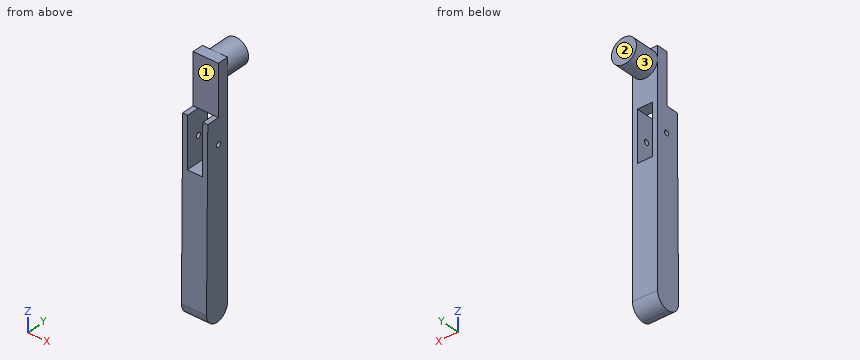
from build123d import *

# Parameters (mm, degrees)
BOSS_EXTRUDE1_DEPTH = 50
BOSS_EXTRUDE2_START = 35.418994
SKETCH2_R           = 25
BOSS_EXTRUDE2_DEPTH = 50
SKETCH4_W           = 30
SKETCH4_H           = 100
CUT_EXTRUDE1_DEPTH  = 318.853328976
SKETCH5_R           = 5
CUT_EXTRUDE2_DEPTH  = 326.310841007


with BuildPart() as part:
    # Sketch1 → Boss-Extrude1 (new body)
    with BuildSketch(Plane(origin=(0, 0, 0), x_dir=(0, 0, -1), z_dir=(1, 0, 0))):
        with BuildLine():
            Line((140.111731844, 35.418994413), (-209.888268156, 35.418994413))
            Line((-209.888268156, 35.418994413), (-309.888268156, 35.418994413))
            Line((-309.888268156, 35.418994413), (-309.888268156, 13.43575419))
            Line((-309.888268156, 13.43575419), (-209.888268156, 13.43575419))
            Line((-209.888268156, 13.43575419), (-209.888268156, -11.56424581))
            Line((-209.888268156, -11.56424581), (139.680798176, -14.577291234))
            ThreePointArc((139.680798176, -14.577291234), (115.112660449, 10.634469251), (140.111731844, 35.418994413))
        make_face()
        with BuildLine():
            Line((140.111731844, -14.581005587), (140.111731844, 35.418994413))
            ThreePointArc((140.111731844, 35.418994413), (115.112660449, 10.634469251), (139.680798176, -14.577291234))
            Line((139.680798176, -14.577291234), (140.111731844, -14.581005587))
        make_face()
        with BuildLine():
            ThreePointArc((165.111731844, 10.418994413), (157.789401373, 28.096663943), (140.111731844, 35.418994413))
            Line((140.111731844, 35.418994413), (140.111731844, -14.581005587))
            ThreePointArc((140.111731844, -14.581005587), (157.789401373, -7.258675116), (165.111731844, 10.418994413))
        make_face()
    extrude(amount=BOSS_EXTRUDE1_DEPTH)

    # Sketch2 → Boss-Extrude2 (add)
    with BuildSketch(Plane(origin=(0, 0, 0), x_dir=(1, 0, 0), z_dir=(0, 1, 0)).offset(BOSS_EXTRUDE2_START)):
        with Locations(Location((25, -284.888268156, 0), (0, 0, 270))):
            Circle(SKETCH2_R)
    extrude(amount=BOSS_EXTRUDE2_DEPTH)

    # Sketch4 → Cut-Extrude1 (cut, through all)
    with BuildSketch(Plane(origin=(0, 35.418994413, 0), x_dir=(1, 0, 0), z_dir=(0, 1, 0))):
        with Locations((25, -159.888268156)):
            Rectangle(SKETCH4_W, SKETCH4_H)
    extrude(amount=-CUT_EXTRUDE1_DEPTH, mode=Mode.SUBTRACT)

    # Sketch5 → Cut-Extrude2 (cut, through all)
    with BuildSketch(Plane(origin=(50, 0, 0), x_dir=(0, 0, -1), z_dir=(1, 0, 0))):
        with Locations((-159.888268156, 13.945126907)):
            Circle(SKETCH5_R)
    extrude(amount=-CUT_EXTRUDE2_DEPTH, mode=Mode.SUBTRACT)


solid = part.part
Geometry check sheet. Reference: the model listing, model coordinates, mm. Face numbers are marked on the shaded views. A direction names the side the tool comes from. Give positions to 0.01 mm unless a question says otherwise; leave off trailing zeros. Write each loop counter-clockwise with the first axis right and the second up, starting at its lowest first coordinate (ties: lowest second). Pieces come first, ordered by that corner, then holes.
1) Go/stop test with flat-tipped pins: pin 1 Ø25 at (x, z) = (37.5, 257) entering from -Y; pin 2 Ø6 at (x, y) = (15.5, 57) entering from -Z; pin 3 Ø5 at (x, y) = (45.5, 0.5) entering from +Z. Record where each tip stops, or that it passes through.
Values follow:
pin 1: stops at y = 13.44
pin 2: stops at z = 260.75
pin 3: stops at z = 209.89
2) Cross-section at B-B (x = 5). Record the boundary of the cut face in (y, z).
Values follow:
outline: (-14.58, -140.11) arc R25 ccw to (35.42, -140.11) - (35.42, 269.89) - (85.42, 269.89) - (85.42, 299.89) - (35.42, 299.89) - (35.42, 309.89) - (13.44, 309.89) - (13.44, 209.89) - (-11.56, 209.89) - close; hole circle Ø10 at (13.95, 159.89)
3) Cross-section at C-C (y = 48). Record the boundary of the cut face in (x, z).
Values follow:
outline: circle Ø50 at (25, 284.89)
4) Cross-section at D-D (z = 13). Record the boundary of the cut face in (x, y), plus the area to 3 significant figures.
Values follow:
outline: (0, -13.26) - (50, -13.26) - (50, 35.42) - (0, 35.42) - close
area: 2,430 mm2
5) Thickness scan on line 1 (X direction, y = 10, z = 177.5); line 2 (Z direction, x = 25, y = 69); line 3 (Y direction, x = 29.5, z = 222). Record the ranges inside material, lowest first.
Values follow:
line 1: x = 0 to 10, 40 to 50
line 2: z = 259.89 to 309.89
line 3: y = 13.44 to 35.42
6) Cross-section at A-A (x = 30). Record the boundary of the cut face in (y, z).
Values follow:
outline: (-14.58, -140.11) arc R25 ccw to (35.42, -140.11) - (35.42, 109.89) - (-12.43, 109.89) - close; (13.44, 209.89) - (35.42, 209.89) - (35.42, 260.39) - (85.42, 260.39) - (85.42, 309.38) - (35.42, 309.38) - (35.42, 309.89) - (13.44, 309.89) - close
7) Set-up check for the marked faces 1, 2 and 3: record each of +Z, -Z, +X, -X, +Y, -Y from which the full face is reachable in a straight line by a thin tool's end or side.
Values follow:
face 1: +Z, +X, -X, -Y
face 2: +Z, -Z, +X, -X, +Y
face 3: +Y
